The listing builds one solid part. Answer for the finished solid, in the listing's coordinates (mm). Face numbers are marked on the shaded views. A direction names the side the tool comes from. Round coordinates to 2 decimals unless told otherwise and drop trailing zeros. Write each loop counter-clockwise with the first axis right and the second up, starting at its lowest first coordinate (ties: lowest second). Pieces come first, ordered by that corner, then holes.
from build123d import *

# Parameters (mm, degrees)
SKETCH1_W                                     = 300
SKETCH1_H                                     = 350
SKETCH1_R                                     = 2.88
ELECTRONICS_TRAY_STRUCTURAL_PANEL_DEPTH       = 1.5
SKETCH2_W                                     = 264
SKETCH2_H                                     = 314
SKETCH2_W_2                                   = 257
SKETCH2_H_2                                   = 307
ELECTRONICS_TRAY_STRUCTURAL_PANEL_INSET_DEPTH = 1.9


with BuildPart() as part:
    # Sketch1 → Electronics tray structural panel (new, symmetric)
    with BuildSketch(Plane(origin=(0, 0, 0), x_dir=(1, 0, 0), z_dir=(0, 1, 0))):
        Rectangle(SKETCH1_W, SKETCH1_H)
        with Locations(Location((140.1, 165.1, 0), (0, 0, 270))):
            Circle(SKETCH1_R, mode=Mode.SUBTRACT)
        with Locations(Location((-140.1, 165.1, 0), (0, 0, 270))):
            Circle(SKETCH1_R, mode=Mode.SUBTRACT)
        with Locations(Location((140.1, -165.1, 0), (0, 0, 270))):
            Circle(SKETCH1_R, mode=Mode.SUBTRACT)
        with Locations(Location((-140.1, -165.1, 0), (0, 0, 270))):
            Circle(SKETCH1_R, mode=Mode.SUBTRACT)
    extrude(amount=ELECTRONICS_TRAY_STRUCTURAL_PANEL_DEPTH, both=True)

    # Sketch2 → Electronics tray structural panel inset stiffener (add, symmetric)
    with BuildSketch(Plane(origin=(0, 0, 0), x_dir=(1, 0, 0), z_dir=(0, 1, 0))):
        Rectangle(SKETCH2_W, SKETCH2_H)
        Rectangle(SKETCH2_W_2, SKETCH2_H_2, mode=Mode.SUBTRACT)
    extrude(amount=ELECTRONICS_TRAY_STRUCTURAL_PANEL_INSET_DEPTH, both=True)


solid = part.part
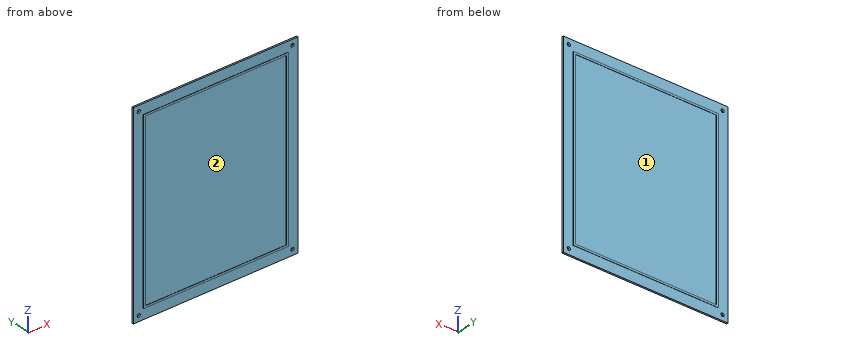
1. Straight lines are drawn through the part: line 1 along Z through (x, y) = (-140.1, 0.35); line 2 along X through (y, z) = (0.8, 165.1); line 3 along Z through (x, y) = (12, 1.7). For each, find the intervals that lie inside material, in ascending order.
Geometry says:
line 1: z = -175 to -167.98, -162.22 to 162.22, 167.98 to 175
line 2: x = -150 to -142.98, -137.22 to 137.22, 142.98 to 150
line 3: z = -157 to -153.5, 153.5 to 157
2. A tool of negligible diameter and unlimited length cuts with its end or side. For the marked faces 1 and 2, from which of +Z, -Z, +X, -X, +Y, -Y can it reach the whole face along a straight path? Write none if from no direction.
Geometry says:
face 1: +Y
face 2: -Y
3. Section A-A on x = 24 is taken. Determine the outline of the cut face in (y, z), plus the area to 3 significant figures.
Geometry says:
outline: (-1.9, -157) - (-1.5, -157) - (-1.5, -175) - (1.5, -175) - (1.5, -157) - (1.9, -157) - (1.9, -153.5) - (1.5, -153.5) - (1.5, 153.5) - (1.9, 153.5) - (1.9, 157) - (1.5, 157) - (1.5, 175) - (-1.5, 175) - (-1.5, 157) - (-1.9, 157) - (-1.9, 153.5) - (-1.5, 153.5) - (-1.5, -153.5) - (-1.9, -153.5) - close
area: 1,060 mm2
4. Given pin 1 (4.5 mm diameter, centred on x = 140.1, z = -165.1, fed in from -Y); pin 2 (2 mm diameter, centred on x = -42, z = -95, fed in from +Y); pin 3 (6.5 mm diameter, centred on x = 140.1, z = 165.1, fed in from -Y), each flat-ended and moving along its own axis, determine where each tip first touches the part or whether it passes through.
Geometry says:
pin 1: passes through
pin 2: stops at y = 1.5
pin 3: stops at y = -1.5
5. Section B-B on z = -67.5 is taken. Determine the outline of the cut face in (x, y).
Geometry says:
outline: (-150, -1.5) - (-132, -1.5) - (-132, -1.9) - (-128.5, -1.9) - (-128.5, -1.5) - (128.5, -1.5) - (128.5, -1.9) - (132, -1.9) - (132, -1.5) - (150, -1.5) - (150, 1.5) - (132, 1.5) - (132, 1.9) - (128.5, 1.9) - (128.5, 1.5) - (-128.5, 1.5) - (-128.5, 1.9) - (-132, 1.9) - (-132, 1.5) - (-150, 1.5) - close
